Read the model definition and answer for the solid it produces. Units are mm, in the model's axes. A direction names the side the tool comes from. Coordinates: 2 decimals unless noted, no trailing zeros. Loops run counter-clockwise (first coordinate to the right, second up) from the corner with the lowest first, then second, coordinate; pieces in that order, holes last. Notation, with made-up numbers: (-25, 34) - (-2, 34) arc R34 cw to (-2, 73) - close; hole circle Ø6 at (38, 7.25). An arc over 180 degrees is marked (long way). Use one line per item in the form item = value. Start each with the question number.
1) The mould has two halves that part along X. Classify faces 3 (the face through (-98, 29, 29)), 4 (the face through (-106, 29, 29)), 5 (the face through (-100, 29, 30)), 6 (the face through (-100.1, 28, 27.8)): released by +X, released by -X, zero draft, split by the parting line, or undercut.
2) A cutting plane is placed at A-A (x = -101.25). Give the vertices of the cut face in (y, z).
3) Consider line 1 (Z direction, x = -100, y = 28.55); line 2 (X direction, y = 29.65, z = 29.5). Determine where each line is inside the solid, lowest interval first.
4) Which of the six approach directions +Z, -Z, +X, -X, +Y, -Y give full straight-line access (tool end or side, diameter ignored) to faces 1 (the face through (-102, 29, 29)), 2 (the face through (-94, 29, 29))?
5) A cutting plane is placed at C-C (z = 29.5). Give the vertices of the cut face in (x, y).
6) A cutting plane is placed at B-B (y = 29.1). Give the vertices of the cut face in (x, z), and give its area (3 significant figures).
from build123d import *

# Parameters (mm, degrees)
BOX013_W     = 4
BOX013_H     = 2
BOX013_DEPTH = 2
BOX012_W     = 12
BOX012_H     = 2
BOX012_DEPTH = 10


with BuildPart() as cube011:
    # Box013 → Box013 (new body)
    with BuildSketch(Plane(origin=(4, 0, 30), x_dir=(1, 0, 0), z_dir=(0, 0, 1))):
        with Locations((2, 1)):
            Rectangle(BOX013_W, BOX013_H)
    extrude(amount=BOX013_DEPTH)


with BuildPart() as obj1:
    # Box012 → Box012 (new body)
    with BuildSketch(Plane.XY.offset(26)):
        with Locations((6, 1)):
            Rectangle(BOX012_W, BOX012_H)
    extrude(amount=BOX012_DEPTH)

    # Cut005: cut Cube011
    add(cube011.part, mode=Mode.SUBTRACT)


with BuildPart() as obj1_1:
    # Cut005 placement: moved
    add(obj1.part.moved(Location((-106, 28, -2))))


solid = obj1_1.part
Found:
q1.face_3 = undercut
q1.face_4 = released by -X
q1.face_5 = undercut
q1.face_6 = zero draft
q2.outline = (28, 24) - (30, 24) - (30, 28) - (28, 28) - close; (28, 30) - (30, 30) - (30, 34) - (28, 34) - close
q3.line_1 = 24 to 28, 30 to 34
q3.line_2 = -106 to -102, -98 to -94
q4.face_1 = +Y, -Y
q4.face_2 = +Z, -Z, +X, +Y, -Y
q5.outline = (-106, 28) - (-102, 28) - (-102, 30) - (-106, 30) - close; (-98, 28) - (-94, 28) - (-94, 30) - (-98, 30) - close
q6.outline = (-106, 24) - (-94, 24) - (-94, 34) - (-106, 34) - close; hole (-102, 28) - (-98, 28) - (-98, 30) - (-102, 30) - close
q6.area = 112 mm^2
